For this review, take the finished solid that the model builds, in its own axes (mm). Coordinates: 2 decimals unless noted, no trailing zeros. Write each loop counter-clockwise with the first axis right and the second up, starting at its lowest first coordinate (ties: lowest second). Pieces come first, ordered by that corner, then holes. Notation, with made-up numbers: M 76.25,44 L 89.25,44 A10 ccw 89.25,53 Z; hole C -21,15 d10. An arc over 180 degrees is marked long. Return JSON: item names as keys, results as strings.
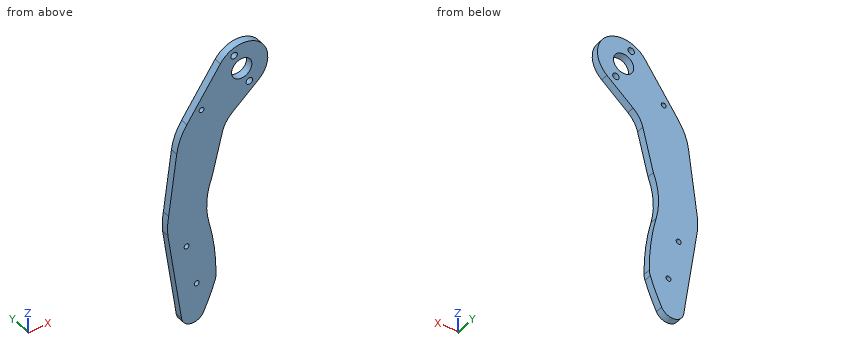
```python
from build123d import *

# Parameters (mm, degrees)
SKETCH1_R                = 7
SKETCH1_R_2              = 1.7
BOSS_EXTRUDE2_DEPTH      = 5
CUT_EXTRUDE1_REACH       = 176.989
SKETCH3_R                = 1.7
M4_CLEARANCE_HOLE1_D     = 4.5
M4_CLEARANCE_HOLE1_DEPTH = 10.1
M4_CLEARANCE_HOLE1_TIP   = 1.351936393


with BuildPart() as part:
    # Sketch1 → Boss-Extrude2 (new body)
    with BuildSketch(Plane(origin=(0, 0, 0), x_dir=(1, 0, 0), z_dir=(0, 1, 0))):
        with BuildLine():
            Line((11.446477506, 13.891657666), (-6.606953629, 28.767362089))
            ThreePointArc((-6.606953629, 28.767362089), (-10.806918693, 33.53614027), (-13.298943796, 39.38171661))
            Line((-13.298943796, 39.38171661), (-20.530174792, 68.49716437))
            ThreePointArc((-20.530174792, 68.49716437), (-24.08112857, 84.393152776), (-22.456551163, 100.599709115))
            ThreePointArc((-22.456551163, 100.599709115), (-18.824269383, 120.221092129), (-17.76802696, 140.147870449))
            ThreePointArc((-17.76802696, 140.147870449), (-17.943181625, 142.067888002), (-18.417828761, 143.936539027))
            ThreePointArc((-18.417828761, 143.936539027), (-22.023480215, 153.489775682), (-26.256294904, 162.782156045))
            ThreePointArc((-26.256294904, 162.782156045), (-34.757388509, 167.168565439), (-41.482617684, 160.365590178))
            Line((-41.482617684, 160.365590178), (-50.932711484, 96.056215067))
            ThreePointArc((-50.932711484, 96.056215067), (-51.118515181, 89.191813761), (-50.383474997, 82.364351257))
            Line((-50.383474997, 82.364351257), (-44.819294227, 40.249739786))
            ThreePointArc((-44.819294227, 40.249739786), (-42.41581584, 30.91866257), (-37.850662253, 22.433081678))
            Line((-37.850662253, 22.433081678), (-14.709041721, -10.375167067))
            ThreePointArc((-14.709041721, -10.375167067), (12.242580486, -13.195424322), (11.446477506, 13.891657666))
        make_face()
        with Locations(Location((0, 0, 0), (0, 0, 270))):
            Circle(SKETCH1_R, mode=Mode.SUBTRACT)
        with Locations(Location((-27.673284612, 16.679008328, 0), (0, 0, 270))):
            Circle(SKETCH1_R_2, mode=Mode.SUBTRACT)
    extrude(amount=BOSS_EXTRUDE2_DEPTH)

    # Sketch3 → Cut-Extrude1 (cut, up to next)
    with BuildSketch(Plane(origin=(0, 5, 0), x_dir=(1, 0, 0), z_dir=(0, 1, 0)), mode=Mode.PRIVATE) as cut_extrude1_sk1:
        with Locations(Location((-31, 140, 0), (0, 0, 270))):
            Circle(SKETCH3_R)
    cut_extrude1_tool1 = extrude(cut_extrude1_sk1.sketch, amount=-CUT_EXTRUDE1_REACH, mode=Mode.PRIVATE) & part.part
    # Sketch3 → Cut-Extrude1 (cut, up to next)
    with BuildSketch(Plane(origin=(0, 5, 0), x_dir=(1, 0, 0), z_dir=(0, 1, 0)), mode=Mode.PRIVATE) as cut_extrude1_sk2:
        with Locations(Location((-38, 110, 0), (0, 0, 270))):
            Circle(SKETCH3_R)
    cut_extrude1_tool2 = extrude(cut_extrude1_sk2.sketch, amount=-CUT_EXTRUDE1_REACH, mode=Mode.PRIVATE) & part.part
    add(cut_extrude1_tool1.solids().sort_by_distance((-31, 5, -140))[0], mode=Mode.SUBTRACT)
    add(cut_extrude1_tool2.solids().sort_by_distance((-38, 5, -110))[0], mode=Mode.SUBTRACT)

    # M4 Clearance Hole1
    with Locations(Plane(origin=(-5.251206507, 5, 11.618404805), x_dir=(0, 0, 1), z_dir=(0, 1, 0))):
        with Locations((0, 0), (-23.23680961, 10.502413014)):
            Hole(M4_CLEARANCE_HOLE1_D / 2, depth=M4_CLEARANCE_HOLE1_DEPTH)
            with Locations((0, 0, -(M4_CLEARANCE_HOLE1_DEPTH + M4_CLEARANCE_HOLE1_TIP / 2))):  # 118° drill point
                Cone(0, M4_CLEARANCE_HOLE1_D / 2, M4_CLEARANCE_HOLE1_TIP, mode=Mode.SUBTRACT)


solid = part.part
```
1. Clearance check with flat-ended pins moving along their axes: pin 1 Ø2.5 at (x, z) = (-27.67, -16.68) entering from +Y; pin 2 Ø5 at (x, z) = (5.25, -11.62) entering from -Y; pin 3 Ø3 at (y, z) = (0.5, -5) entering from -X. State where each tip first meets the part, or that it passes through.
Checks:
{"pin 1": "through", "pin 2": "y = 0", "pin 3": "x = -26.61"}
2. We need section B-B (x = 0). State the section outline as (y, z) points.
Checks:
{"outline": "M 0,-23.32 L 5,-23.32 L 5,-7 L 0,-7 Z; M 0,7 L 5,7 L 5,18 L 0,18 Z"}
3. We need section C-C (y = 3.8). State the section outline as (x, z) points, plus the area to 3 significant figures.
Checks:
{"outline": "M -50.93,-96.06 L -41.48,-160.37 A8.08 ccw -26.26,-162.78 A153.5 ccw -18.42,-143.94 A12.23 ccw -17.77,-140.15 A153.5 ccw -22.46,-100.6 A51.17 cw -20.53,-68.5 L -13.3,-39.38 A20 cw -6.61,-28.77 L 11.45,-13.89 A18 ccw long -14.71,10.38 L -37.85,-22.43 A40 ccw -44.82,-40.25 L -50.38,-82.36 A51.17 ccw Z; hole C -38,-110 d3.4; hole C -31,-140 d3.4; hole C -27.67,-16.68 d3.4; hole C -5.25,11.62 d4.5; hole C 0,0 d14; hole C 5.25,-11.62 d4.5", "area": "5,210 mm2"}
4. We need section A-A (z = -110). State the section outline as (x, y) points.
Checks:
{"outline": "M -48.88,0 L -39.7,0 L -39.7,5 L -48.88,5 Z; M -36.3,0 L -20.39,0 L -20.39,5 L -36.3,5 Z"}
5. Wall thickness on L1, parallel to Z at x = 5.5, y = 2.55; L2, parallel to Z at x = 4, y = 2.85; L3, parallel to Z at x = -39, y = 2.3: over which ranges is each line inside the solid? List them lowest first. Write a range as from..to.
Checks:
{"L1": "-18.79..-13.85, -9.38..-4.33, 4.33..17.14", "L2": "-20.03..-13.49, -9.75..-5.74, 5.74..17.55", "L3": "-165.1..-111.37, -108.63..-24.16"}
6. We need section D-D (x = -10). State the section outline as (y, z) points, plus the area to 3 significant figures.
Checks:
{"outline": "M 0,-32.35 L 5,-32.35 L 5,14.97 L 0,14.97 Z", "area": "237 mm2"}
